```python
from build123d import *

# Parameters (mm, degrees)
F0_R      = 11
F1_DEPTH  = 150
F2_R      = 20
F3_DEPTH  = 7.9
F4_R      = 11
F5_DEPTH  = 3.1
F6_R      = 10
F7_DEPTH  = 6
F8_R      = 11
F9_DEPTH  = 11
F11_D     = 10.3
F11_DEPTH = 35
F11_TIP   = 3.094432188
F12_SIZE  = 1
F13_SIZE  = 0.5


with BuildPart() as f1:
    # F0 (on Top) → F1 (new body)
    with BuildSketch(Plane.XY):
        Circle(F0_R)
    extrude(amount=F1_DEPTH)

    # F2 (on face) → F3 (join)
    with BuildSketch(Plane.XY.offset(150)):
        Circle(F2_R)
    extrude(amount=F3_DEPTH)

    # F4 (on face) → F5 (join)
    with BuildSketch(Plane.XY.offset(157.9)):
        Circle(F4_R)
    extrude(amount=F5_DEPTH)

    # F6 (on face) → F7 (join)
    with BuildSketch(Plane.XY.offset(161)):
        Circle(F6_R)
    extrude(amount=F7_DEPTH)

    # F8 (on face) → F9 (join)
    with BuildSketch(Plane.XY.offset(167)):
        Circle(F8_R)
    extrude(amount=F9_DEPTH)

    # F11
    with Locations(Plane(origin=(0, 0, 0), x_dir=(1, 0, 0), z_dir=(0, 0, -1))):
        with Locations((0, 0)):
            Hole(F11_D / 2, depth=F11_DEPTH)
            with Locations((0, 0, -(F11_DEPTH + F11_TIP / 2))):  # 118° drill point
                Cone(0, F11_D / 2, F11_TIP, mode=Mode.SUBTRACT)

    # F12
    f12_edges = [f1.edges().sort_by_distance(p)[0] for p in [
        (-11, 0, 0),
        (-5.15, 0, 0),
    ]]
    chamfer(f12_edges, length=F12_SIZE)

    # F13
    f13_edges = [f1.edges().sort_by_distance(p)[0] for p in [
        (-20, 0, 150),
        (-20, 0, 157.9),
        (-11, 0, 161),
        (-11, 0, 167),
        (-11, 0, 178),
    ]]
    chamfer(f13_edges, length=F13_SIZE)


solid = f1.part
```
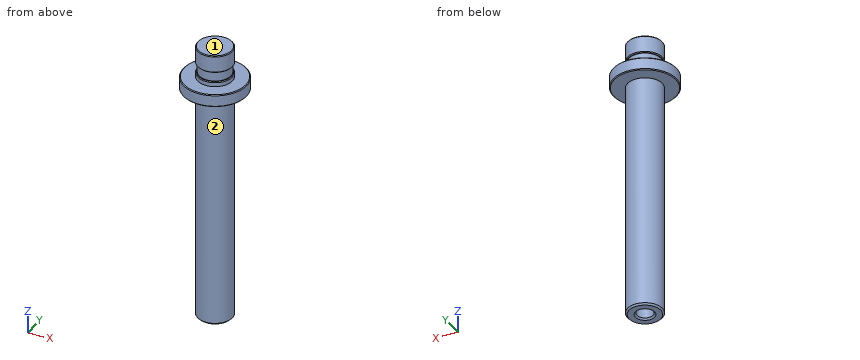
Model file for the job. Use its own axes, mm. Face numbers are marked on the shaded views. A direction names the side the tool comes from. Coordinates: 2 decimals unless noted, no trailing zeros. Order: outer loops, then holes, each group sorted by start corner. A loop starts at its lowest first (then second) coordinate and runs counter-clockwise, first axis right, second up. Notation, with made-up numbers: (83, 23.25) - (121, 23.25) arc R26 cw to (121, 57.25) - close; hole circle Ø5 at (5, -27.75). An arc over 180 degrees is marked (long way). Return JSON: item names as keys, results as strings. Group by question number.
1) Saw through at C-C, the plane z = 164. Write the cut outline in (x, y).
2) Saw through at A-A, the plane z = 103. Write the cut outline in (x, y), plus the area to 3 significant figures.
3) Probe line 1 (Y direction, x = 0, z = 23); line 2 (Y direction, x = 0, z = 156); line 3 (Z direction, x = 0.5, y = 14). List the from-to ranges inside material, lowest first. Write a range as from..to.
4) Saw through at B-B, the plane z = 11. Write the cut outline in (x, y), plus the area to 3 significant figures.
5) Flat gauge pins, fed straight in: P1, Ø1, axis at x = 6, z = 72, coming from the +Y side; P2, Ø6, axis at x = 0, y = 0, coming from the -Z side; P3, Ø10, axis at y = 2.5, z = 23, coming from the +X side. Where does each tip first touch, or does it go through?
6) Tool access for the marked faces 1 and 2: list every direction of +Z, -Z, +X, -X, +Y, -Y with a clear straight run to the whole face (end or side of a thin tool).
Values found:
{
 "1": {"outline": "circle Ø20 at (0, 0)"},
 "2": {"outline": "circle Ø22 at (0, 0)", "area": "380 mm²"},
 "3": {"line 1": "y = -11..-5.15, 5.15..11", "line 2": "y = -20..20", "line 3": "z = 150..157.9"},
 "4": {"outline": "circle Ø22 at (0, 0); hole circle Ø10.3 at (0, 0)", "area": "297 mm²"},
 "5": {"P1": "stops at y = 9.53", "P2": "stops at z = 36.29", "P3": "stops at x = 11"},
 "6": {"face 1": "+Z, +X, -X, +Y, -Y", "face 2": "-Z"}
}
